from build123d import *

# Parameters (mm, degrees)
CUT_EXTRUDE_1_DEPTH = 14.7
SKETCH_4_W          = 25
SKETCH_4_H          = 39.508434057
SKETCH_4_R          = 2.5
EXTRUDE_1_DEPTH     = 0.12
CHAMFER_1_SIZE      = 5
FILLET_1_R          = 2


with BuildPart() as part:
    # 草图2 → 旋转1 (revolve)
    with BuildSketch(Plane(origin=(0, 0, 0), x_dir=(1, 0, 0), z_dir=(0, 1, 0)), mode=Mode.PRIVATE) as revolve_1_sk:
        Polygon((3.1, 15.75), (20, 15.75), (20, 12.5), (16.5, 12.5), (16.5, -12.5), (20, -12.5), (20, -15.75), (3.1, -15.75), align=None)
    revolve(revolve_1_sk.sketch.rotate(Axis((0, 0, -15.75), (0, 0, 1)), 180), axis=Axis((0, 0, -15.75), (0, 0, 1)))

    # 草图3 → 切除-拉伸1 (cut)
    with BuildSketch(Plane.XY.offset(15.75)):
        with BuildLine():
            Line((-0.7, 5.455272679), (-0.7, 11.979565935))
            ThreePointArc((-0.7, 11.979565935), (-10.392304845, 6), (-10.724608426, -5.383565185))
            Line((-10.724608426, -5.383565185), (-5.074404724, -2.121418557))
            ThreePointArc((-5.074404724, -2.121418557), (-4.763139721, 2.75), (-0.7, 5.455272679))
        make_face()
        with BuildLine():
            Line((-4.374404724, -3.333854122), (-10.024608426, -6.59600075))
            ThreePointArc((-10.024608426, -6.59600075), (0, -12), (10.024608426, -6.59600075))
            Line((10.024608426, -6.59600075), (4.374404724, -3.333854122))
            ThreePointArc((4.374404724, -3.333854122), (0, -5.5), (-4.374404724, -3.333854122))
        make_face()
        with BuildLine():
            ThreePointArc((12, 0), (8.729261137, 8.23407554), (0.7, 11.979565935))
            Line((0.7, 11.979565935), (0.7, 5.455272679))
            ThreePointArc((0.7, 5.455272679), (4.129164564, 3.633180425), (5.5, 0))
            ThreePointArc((5.5, 0), (5.392551622, -1.081844262), (5.074404724, -2.121418557))
            Line((5.074404724, -2.121418557), (10.724608426, -5.383565185))
            ThreePointArc((10.724608426, -5.383565185), (11.676799671, -2.766288026), (12, 0))
        make_face()
    cut_extrude_1 = extrude(amount=-CUT_EXTRUDE_1_DEPTH, mode=Mode.SUBTRACT)

    # 镜向2: 切除-拉伸1 across plane
    add(cut_extrude_1.mirror(Plane.XY), mode=Mode.SUBTRACT)

    # 草图4 → 凸台-拉伸1 (add)
    with BuildSketch(Plane.ZY.offset(16.5)):
        with Locations((0, -19.754217029)):
            Rectangle(SKETCH_4_W, SKETCH_4_H)
        with Locations((7.5, -31.508434057)):
            Circle(SKETCH_4_R, mode=Mode.SUBTRACT)
        with Locations((-7.5, -31.508434057)):
            Circle(SKETCH_4_R, mode=Mode.SUBTRACT)
    extrude(amount=-EXTRUDE_1_DEPTH)

    # 倒角1
    chamfer_1_edges = [part.edges().sort_by_distance(p)[0] for p in [
        (-16.44, -39.508434057, 12.5),
        (-16.44, -39.508434057, -12.5),
    ]]
    chamfer(chamfer_1_edges, length=CHAMFER_1_SIZE)

    # 圆角1
    fillet_1_edges = [part.edges().sort_by_distance(p)[0] for p in [
        (-16.44, -34.508434057, -12.5),
        (-16.44, -39.508434057, 7.5),
        (-16.44, -39.508434057, -7.5),
        (-16.44, -34.508434057, 12.5),
    ]]
    fillet(fillet_1_edges, radius=FILLET_1_R)


solid = part.part
Could you check a few things on this model? Use its own coordinates, in mm. A direction names the side the tool comes from. Give positions to 0.01 mm unless a question says otherwise; leave off trailing zeros. Order: outer loops, then holes, each group sorted by start corner. A loop starts at its lowest first (then second) coordinate and runs counter-clockwise, first axis right, second up. Notation, with made-up numbers: (-37.75, -3) -> (0.25, -3) arc R13 cw to (0.25, 9) -> close; hole circle Ø5 at (88, -38). An arc over 180 degrees is marked (long way). Answer in a Markdown table with one row per item. Add a question column.
Item 1: Please list where these lines run through material, in increasing order: probe 1 along Z at (x, y) = (-13, 13); probe 2 along Y at (x, z) = (-6.5, 6); probe 3 along Y at (x, z) = (-2, 14).
Item 2: I'm going to push flat-ended pins straight in: P1, Ø1.5, axis at x = -9, z = -10.5, coming from the -Y side; P2, Ø10, axis at x = 15, z = -0.5, coming from the -Y side; P3, Ø5, axis at y = 9, z = -4.5, coming from the -X side; P4, Ø9, axis at x = 4.5, y = 6, coming from the -Z side. Where does each tip first touch, or does it pass through?
Item 3: Imagine slicing it at D-D (x = -14). List the corners of the cut face in (y, z) for me, and give its area (3 significant figures).
Item 4: We'd pull the mould along Z, two halves only. Please class faces 4 (the flat face through (0, -8, -1.05)), 5 (the flat face through (0.7, 9, 9)), 6 (the flat face through (-2.9, -16.4, -12.5)): pulls with the +Z half, pulls with the -Z half, needs draft (parallel to the pull), parting line crosses it, or undercut.
Item 5: Imagine slicing it at C-C (y = -8). List the corners of the cut face in (x, z) for me.
Item 6: For faces 1 (the flat face through (-7.939, -3.775, -8.503)), 2 (the flat face through (0, -8, 1.05)), 3 (the flat face through (0, 4, -15.75)), which set-ups out of +Z, -Z, +X, -X, +Y, -Y let a thin tool reach every point of the face, with its end or its side?
Item 7: Imagine slicing it at B-B (x = 0). List the corners of the cut face in (y, z) for me, and give its area (3 significant figures).
Item 8: Imagine slicing it at A-A (z = -3.5). List the corners of the cut face in (x, y) for me.
Result:
| question | item | result |
|---|---|---|
| 1 | probe 1 | -15.75 to -12.5, 12.5 to 15.75 |
| 1 | probe 2 | -15.17 to -10.09, -4.56 to -2.94, 10.09 to 15.17 |
| 1 | probe 3 | -19.9 to -11.83, -5.12 to -2.37, 2.37 to 5.12, 11.83 to 19.9 |
| 2 | P1 | y = -14.29 |
| 2 | P2 | y = -13.12 |
| 2 | P3 | x = -15.17 |
| 2 | P4 | z = -15.75 |
| 3 | outline | (-14.28, -15.75) -> (14.28, -15.75) -> (14.28, -12.5) -> (8.73, -12.5) -> (8.73, 12.5) -> (14.28, 12.5) -> (14.28, 15.75) -> (-14.28, 15.75) -> (-14.28, 12.5) -> (-8.73, 12.5) -> (-8.73, -12.5) -> (-14.28, -12.5) -> close |
| 3 | area | 622 mm2 |
| 4 | face 4 | pulls with the -Z half |
| 4 | face 5 | needs draft |
| 4 | face 6 | undercut |
| 5 | outline | (-18.33, -15.75) -> (-8.94, -15.75) -> (-8.94, -1.05) -> (8.94, -1.05) -> (8.94, -15.75) -> (18.33, -15.75) -> (18.33, -12.5) -> (14.43, -12.5) -> (14.43, 12.5) -> (18.33, 12.5) -> (18.33, 15.75) -> (8.94, 15.75) -> (8.94, 1.05) -> (-8.94, 1.05) -> (-8.94, 15.75) -> (-18.33, 15.75) -> (-18.33, 12.5) -> (-16.5, 12.5) -> (-16.5, -12.5) -> (-18.33, -12.5) -> close; hole (-16.38, -12.5) -> (-14.43, -12.5) -> (-14.43, 12.5) -> (-16.38, 12.5) -> close |
| 6 | face 1 | -Z |
| 6 | face 2 | +Z |
| 6 | face 3 | -Z, +X, -X, +Y, -Y |
| 7 | outline | (-20, -15.75) -> (-12, -15.75) -> (-12, -1.05) -> (-5.5, -1.05) -> (-5.5, -15.75) -> (-3.1, -15.75) -> (-3.1, 15.75) -> (-5.5, 15.75) -> (-5.5, 1.05) -> (-12, 1.05) -> (-12, 15.75) -> (-20, 15.75) -> (-20, 12.5) -> (-16.5, 12.5) -> (-16.5, -12.5) -> (-20, -12.5) -> close; (3.1, -15.75) -> (20, -15.75) -> (20, -12.5) -> (16.5, -12.5) -> (16.5, 12.5) -> (20, 12.5) -> (20, 15.75) -> (3.1, 15.75) -> close |
| 7 | area | 699 mm2 |
| 8 | outline | (-16.5, -39.51) -> (-16.38, -39.51) -> (-16.38, -1.99) arc R16.5 ccw (long way) to (-16.5, 0) -> close; hole (-10.72, -5.38) -> (-5.07, -2.12) arc R5.5 cw to (-0.7, 5.46) -> (-0.7, 11.98) arc R12 ccw to start; hole (-10.02, -6.6) arc R12 ccw to (10.02, -6.6) -> (4.37, -3.33) arc R5.5 cw to (-4.37, -3.33) -> close; hole circle Ø6.2 at (0, 0); hole (0.7, 5.46) arc R5.5 cw to (5.07, -2.12) -> (10.72, -5.38) arc R12 ccw to (0.7, 11.98) -> close |
